Autodesk Inventor part; units mm, degrees
ref_plane "YZ Plane" through (0, 0, 0) normal (1, 0, 0) x (0, 1, 0)
ref_plane "XZ Plane" through (0, 0, 0) normal (0, 1, 0) x (-1, 0, 0)
ref_plane "XY Plane" through (0, 0, 0) normal (0, 0, 1) x (1, 0, 0)
sketch "Sketch1" plane through (0, 0, 0) normal (0, 0, 1) x (1, 0, 0)
  line L0 (-203.2, -25.4) -> (203.2, -25.4) construction
  line L1 (203.2, -25.4) -> (203.2, 25.4) construction
  line L2 (203.2, 25.4) -> (-203.2, 25.4) construction
  line L3 (-203.2, 25.4) -> (-203.2, -25.4) construction
  line L4 (-203.2, -25.4) -> (203.2, 25.4) construction
  line L5 (203.2, -25.4) -> (-203.2, 25.4) construction
  circle A0 centre (-164.3694, 123.6318) radius 14.2875 construction
  circle A1 centre (51.4372, 117.2818) radius 14.2875 construction
  line L6 (-157.3708, -518.3539) -> (-157.3708, -1127.9539) construction
  line L7 (-157.3708, -1127.9539) -> (29.9542, -1127.9539) construction
  line L8 (29.9542, -1127.9539) -> (29.9542, -518.3539) construction
  line L9 (29.9542, -518.3539) -> (-157.3708, -518.3539) construction
  line L10 (-164.3694, 123.6318) -> (51.4372, 117.2818) construction
  circle A2 centre (177.8, 0) radius 14.2875
  line L11 (203.2, -25.4) -> (152.4, -25.4)
  line L12 (203.2, -25.4) -> (203.2, 138.2272)
  line L13 (152.4, -25.4) -> (152.4, 88.9)
  line L14 (152.4, 88.9) -> (-203.2, 99.3634)
  line L15 (-203.2, 99.3634) -> (-201.7059, 150.1414)
  line L16 (-201.7059, 150.1414) -> (203.2, 138.2272)
  point P0 (0, 0)
  point P1 (-203.2, 0)
  point P2 (203.2, 0)
  dimension "d0" = 406.4
  dimension "d1" = 50.8
  dimension "d2" = 28.575
  dimension "d3" = 28.575
  dimension "d4" = 187.325
  dimension "d5" = 609.6
  dimension "d6" = 215.9
  dimension "d7" = 6.35
  dimension "d10" = 28.575
  dimension "d11" = 25.4
  dimension "d21" = 50.8
  dimension "d22" = 25.4
  dimension "d23" = 38.1
  dimension "d24" = 114.3
  dimension "d25" = 50.8
extrude "Extrusion1" add sketch "Sketch1" against normal blind 6.35
hole "Hole1" at (51.4372, 117.2818, 0) at (-164.3694, 123.6318, 0) direction (0, 0, -1) diameter 5.1054 end through all
properties part number "CL2-004" material "Aluminum 6061"
Build history of the part. All positions in model axes, mm. Round coordinates to 2 decimals unless told otherwise and drop trailing zeros. Order: outer loops, then holes, each group sorted by start corner. A loop starts at its lowest first (then second) coordinate and runs counter-clockwise, first axis right, second up. Notation, with made-up numbers: (77, -1) - (105, -1) arc R21 cw to (105, 19) - close; hole circle Ø8 at (1, 54). An arc over 180 degrees is marked (long way). Use a Markdown table: item, result.
1) Saw through at D-D on y = 21. Write the cut outline in (x, z).
Recorded:
| item | result |
|---|---|
| outline | (152.4, -6.35) - (203.2, -6.35) - (203.2, 0) - (152.4, 0) - close |
2) Wall check: L1, parallel to X at y = 57.5, z = -4.5; L2, parallel to X at y = -4, z = -4; L3, parallel to Y at x = 177.8, z = -2. Give the ranges that are in metal, low to high.
Recorded:
| item | result |
|---|---|
| L1 | x = 152.4 to 203.2 |
| L2 | x = 152.4 to 164.08, 191.52 to 203.2 |
| L3 | y = -25.4 to -14.29, 14.29 to 138.97 |
3) Saw through at C-C on z = -5. Write the cut outline in (x, y) (1 decimal), and give its area (3 significant figures).
Recorded:
| item | result |
|---|---|
| outline | (-203.2, 99.4) - (152.4, 88.9) - (152.4, -25.4) - (203.2, -25.4) - (203.2, 138.2) - (-201.7, 150.1) - close; hole circle Ø5.1 at (-164.4, 123.6); hole circle Ø5.1 at (51.4, 117.3); hole circle Ø28.6 at (177.8, 0) |
| area | 25,700 mm² |
4) Pull direction X, two halves, no side cores. Call faces 1 (the face through (-3, 103, -6.35)), 2 (the face through (191, -5.47, -3.13)): pulls with the +X half, pulls with the -X half, needs draft (parallel to the pull), parting line crosses it, or undercut.
Recorded:
| item | result |
|---|---|
| face 1 | needs draft |
| face 2 | undercut |
5) Flat gauge pin, fed straight in: pin 1 Ø1 at (x, z) = (-130, -1.5) entering from +Y. Where does the tip first touch, or does it go through?
Recorded:
| item | result |
|---|---|
| pin 1 | stops at y = 148.05 |
6) Saw through at B-B on x = 177.8. Write the cut outline in (y, z).
Recorded:
| item | result |
|---|---|
| outline | (-25.4, -6.35) - (-14.29, -6.35) - (-14.29, 0) - (-25.4, 0) - close; (14.29, -6.35) - (138.97, -6.35) - (138.97, 0) - (14.29, 0) - close |
7) Saw through at A-A on y = 0. Write the cut outline in (x, z).
Recorded:
| item | result |
|---|---|
| outline | (152.4, -6.35) - (163.51, -6.35) - (163.51, 0) - (152.4, 0) - close; (192.09, -6.35) - (203.2, -6.35) - (203.2, 0) - (192.09, 0) - close |
